Drawing for the job (mm, zero at the part's lowest x, y, z). A direction names the side the tool comes from. Coordinates: 2 decimals unless noted, no trailing zeros. Loops run counter-clockwise (first coordinate to the right, second up) from the corner with the lowest first, then second, coordinate; pieces in that order, holes last. Notation, with made-up numbers: (-32, 44) -> (21, 44) arc R21 ccw to (21, 56) -> close; hole circle Ø8 at (16, -3.75). An arc over 180 degrees is marked (long way). Write item = value, one per line. Start each with the question number.
(1) Drill centre lines: line 1 (X direction, y = 11.75, z = 56); line 2 (X direction, y = 15.5, z = 68); line 3 (X direction, y = 17.25, z = 98.5). Where is each one in solid material? Low to high. Write a range as from..to.
(2) Flat gauge pin, fed straight in: P1, Ø2.5, axis at y = 13.5, z = 34, coming from the -X side. Where does the tip first touch, or does it go through?
(3) Pull direction Z, two halves, no side cores. Call the marked faces 1, 2, 3 and 4: +Z half, -Z half, draft (parallel to the pull), parting line (faces both ways), or undercut.
(4) Tool access for the marked faces 5 and 6: list every direction of +Z, -Z, +X, -X, +Y, -Y with a clear straight run to the whole face (end or side of a thin tool).
(5) Band-saw the part on A-A (z = 57.15). Count the separate pieces of the cut face and the enclosed holes in it.
(6) Band-saw the part on B-B (x = 17.5). Write the cut outline in (y, z) (1 decimal), and give its area (3 significant figures).
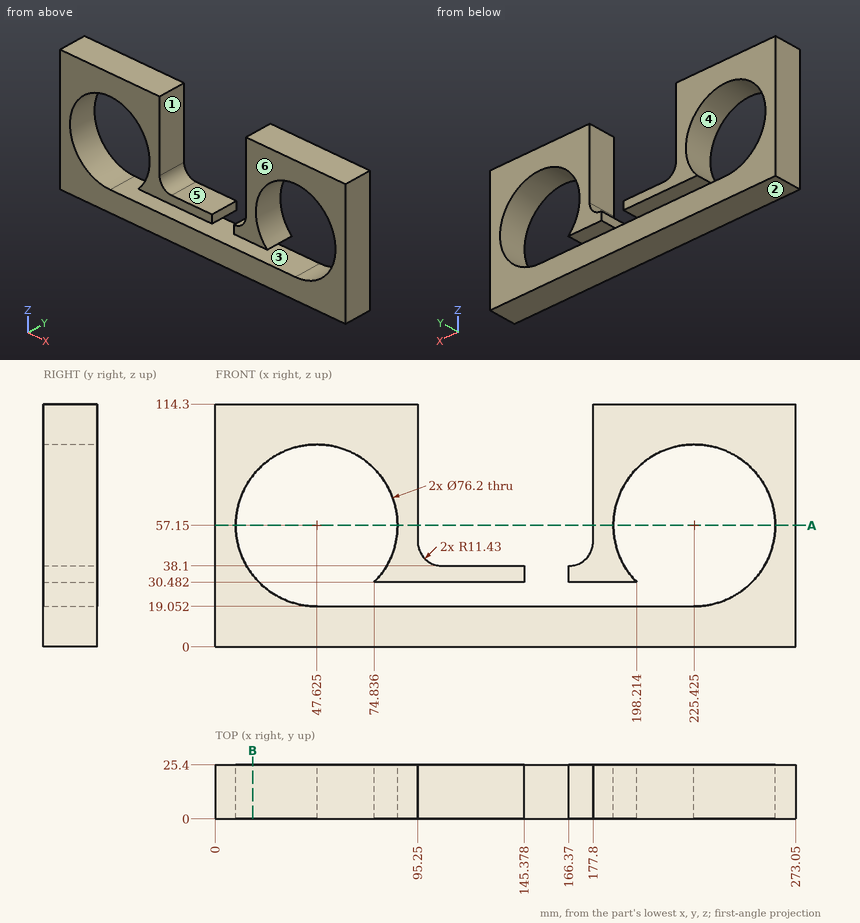
Findings below:
q1.line_1 = 0..9.54, 85.71..95.25, 177.8..187.34, 263.51..273.05
q1.line_2 = 0..11.1, 84.15..95.25, 177.8..188.9, 261.95..273.05
q1.line_3 = 0..95.25, 177.8..273.05
q2.P1 = 0
q3.face_1 = draft
q3.face_2 = -Z half
q3.face_3 = undercut
q3.face_4 = undercut
q4.face_5 = +Z, +Y, -Y
q4.face_6 = +Z, -Z, +X, -X, -Y
q5.separate_pieces = 4
q5.enclosed_holes = 0
q6.outline = (0, 0) -> (25.4, 0) -> (25.4, 33.8) -> (0, 33.8) -> close; (0, 80.5) -> (25.4, 80.5) -> (25.4, 114.3) -> (0, 114.3) -> close
q6.area = 1,720 mm²
